The drawing under review shows one solid part. Ordinate dimensions are in mm from its lowest x, y, z. A direction names the side the tool comes from. Give positions to 0.01 mm unless a question says otherwise; leave off trailing zeros. Write each loop counter-clockwise with the first axis right and the second up, starting at its lowest first coordinate (ties: lowest second). Pieces come first, ordered by that corner, then holes. Notation, with made-up numbers: (40, 6) -> (71, 6) arc R37 cw to (71, 44) -> close; hole circle Ø4 at (21.25, 52). An arc over 180 degrees is marked (long way). Put each result on its own line as item: value. Start each with the question number.
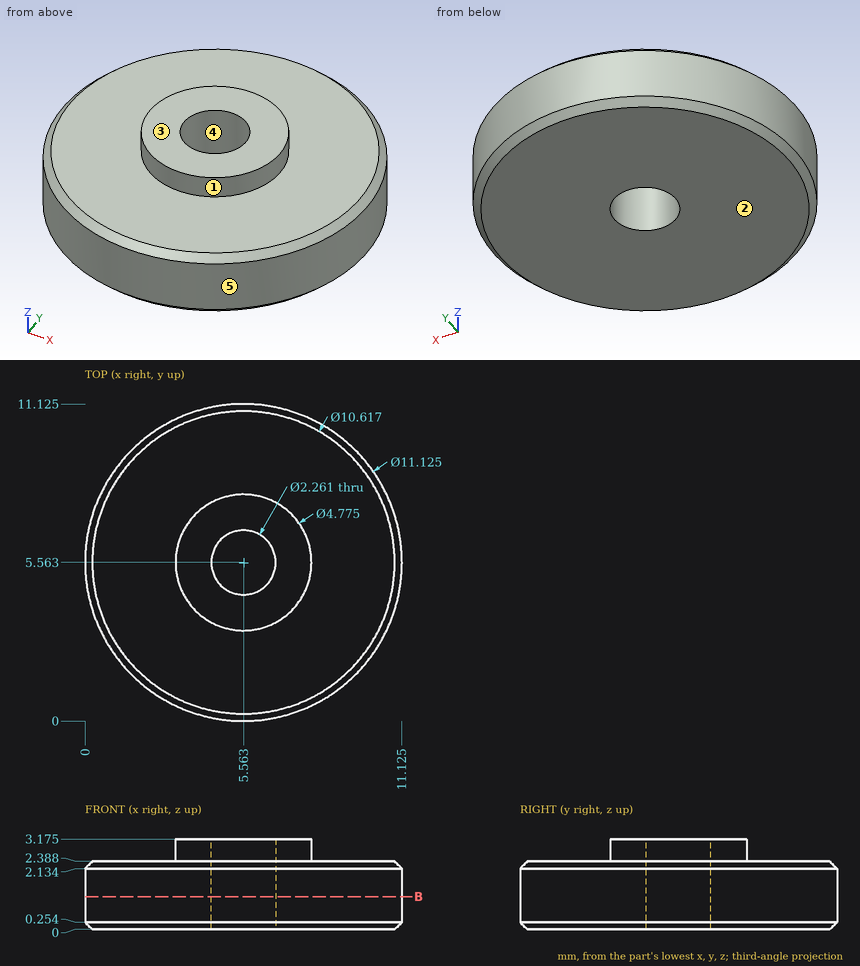
Q1. To check wall thickness, follow probe 1 along X at (y, z) = (5.5, 1.4) (1 decimal); probe 2 along Z at (x, y) = (7.75, 9); probe 3 along Y at (x, z) = (5.75, 2.85). State the ranges of each line that lie inside material, in increasing order. Write a range as from..to.
Q2. Mouldability with a two-part tool opening along X and no side actions: class the marked faces 3, 4 and 5 as +X half, -X half, draft (parallel to the pull), parting line (faces both ways), or undercut.
Q3. Take a section at B-B on z = 1.15. Give the boundary of the cut face in (x, y) (1 decimal), then the cut area to 3 significant figures.
Q4. Machinability: for the marked faces 1 and 2, which of the approach directions +Z, -Z, +X, -X, +Y, -Y give a long, thin tool a straight path to every point of the face, cutting with its end or side? Answer none if there is none.
Q5. For pin 1 (1.5 mm diameter, centred on y = 3.5, z = 2.5, fed in from -X); pin 2 (1.5 mm diameter, centred on x = 3.5, z = 1.5, fed in from +Y); pin 3 (1 mm diameter, centred on y = 2.5, z = 2.5, fed in from -X), all flat-tipped, find the tip position at first contact; note any pin that passes through.
Result:
1. probe 1: x = 0..4.4, 6.7..11.1
1. probe 2: z = 0..2.39
1. probe 3: y = 3.18..4.45, 6.68..7.94
2. face 3: draft
2. face 4: undercut
2. face 5: parting line
3. outline: circle Ø11.1 at (5.6, 5.6); hole circle Ø2.3 at (5.6, 5.6)
3. area: 93.2 mm^2
4. face 1: +Z
4. face 2: -Z, +X, -X, +Y, -Y
5. pin 1: stops at x = 0.18
5. pin 2: stops at y = 10.97
5. pin 3: stops at x = 0.71
